CAD build for the part. Positions are in the model's coordinates, mm. Face numbers are marked on the shaded views. A direction names the side the tool comes from. Give positions to 0.01 mm unless a question says otherwise; leave off trailing zeros. Write each loop counter-clockwise with the first axis right and the second up, starting at its lowest first coordinate (ties: lowest second). Pieces come first, ordered by that corner, then holes. Notation, with made-up numbers: (-13.5, 39.5) -> (39.5, 39.5) arc R26 cw to (39.5, 57.5) -> close; hole circle Ø10 at (-31, 49). An arc over 180 degrees is marked (long way). Answer as a JSON object with one key per item and string values.
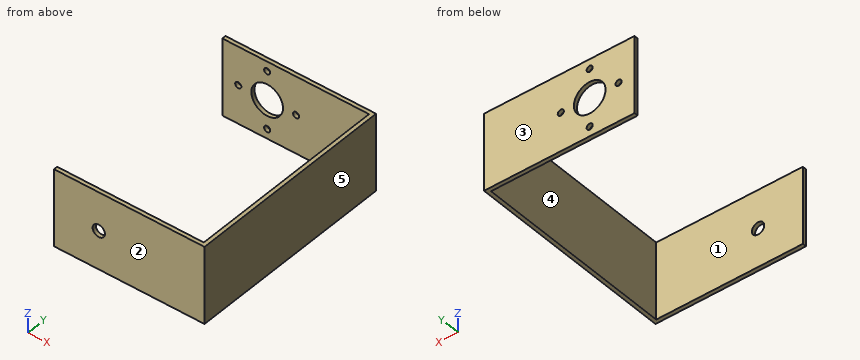
```python
from build123d import *

# Parameters (mm, degrees)
SKETCH_1_W          = 20
SKETCH_1_H          = 54.5
EXTRUDE_1_DEPTH     = 1
SKETCH_2_W          = 20
SKETCH_2_H          = 1
EXTRUDE_2_DEPTH     = 38
SKETCH_3_W          = 20
SKETCH_3_H          = 1
EXTRUDE_3_DEPTH     = 38
SKETCH_4_R          = 4.1
CUT_EXTRUDE_1_DEPTH = 1
SKETCH_5_R          = 0.79
CUT_EXTRUDE_2_DEPTH = 1
SKETCH_6_R          = 0.79
CUT_EXTRUDE_3_DEPTH = 1
SKETCH_7_R          = 0.79
CUT_EXTRUDE_4_DEPTH = 1
SKETCH_8_R          = 0.79
CUT_EXTRUDE_5_DEPTH = 1
SKETCH_9_R          = 1.6
CUT_EXTRUDE_6_DEPTH = 1


with BuildPart() as part:
    # ｽｹｯﾁ1 → ﾎﾞｽ - 押し出し1 (new body)
    with BuildSketch(Plane(origin=(0, 0, 0), x_dir=(0, 0, -1), z_dir=(1, 0, 0))):
        with Locations((10, 27.25)):
            Rectangle(SKETCH_1_W, SKETCH_1_H)
    extrude(amount=EXTRUDE_1_DEPTH)

    # ｽｹｯﾁ2 → ﾎﾞｽ - 押し出し2 (add)
    with BuildSketch(Plane.ZY):
        with Locations((-10, 54)):
            Rectangle(SKETCH_2_W, SKETCH_2_H)
    extrude(amount=EXTRUDE_2_DEPTH)

    # ｽｹｯﾁ3 → ﾎﾞｽ - 押し出し3 (add)
    with BuildSketch(Plane.ZY):
        with Locations((-10, 0.5)):
            Rectangle(SKETCH_3_W, SKETCH_3_H)
    extrude(amount=EXTRUDE_3_DEPTH)

    # ｽｹｯﾁ4 → ｶｯﾄ - 押し出し1 (cut)
    with BuildSketch(Plane(origin=(0, 54.5, 0), x_dir=(1, 0, 0), z_dir=(0, 1, 0))):
        with Locations((-26.39, 10)):
            Circle(SKETCH_4_R)
    extrude(amount=-CUT_EXTRUDE_1_DEPTH, mode=Mode.SUBTRACT)

    # ｽｹｯﾁ5 → ｶｯﾄ - 押し出し2 (cut)
    with BuildSketch(Plane(origin=(0, 54.5, 0), x_dir=(1, 0, 0), z_dir=(0, 1, 0))):
        with Locations((-33.88, 10)):
            Circle(SKETCH_5_R)
    extrude(amount=-CUT_EXTRUDE_2_DEPTH, mode=Mode.SUBTRACT)

    # ｽｹｯﾁ6 → ｶｯﾄ - 押し出し3 (cut)
    with BuildSketch(Plane(origin=(0, 54.5, 0), x_dir=(1, 0, 0), z_dir=(0, 1, 0))):
        with Locations((-18.9, 10)):
            Circle(SKETCH_6_R)
    extrude(amount=-CUT_EXTRUDE_3_DEPTH, mode=Mode.SUBTRACT)

    # ｽｹｯﾁ7 → ｶｯﾄ - 押し出し4 (cut)
    with BuildSketch(Plane(origin=(0, 54.5, 0), x_dir=(1, 0, 0), z_dir=(0, 1, 0))):
        with Locations((-26.39, 2.51)):
            Circle(SKETCH_7_R)
    extrude(amount=-CUT_EXTRUDE_4_DEPTH, mode=Mode.SUBTRACT)

    # ｽｹｯﾁ8 → ｶｯﾄ - 押し出し5 (cut)
    with BuildSketch(Plane(origin=(0, 54.5, 0), x_dir=(1, 0, 0), z_dir=(0, 1, 0))):
        with Locations((-26.39, 17.49)):
            Circle(SKETCH_8_R)
    extrude(amount=-CUT_EXTRUDE_5_DEPTH, mode=Mode.SUBTRACT)

    # ｽｹｯﾁ9 → ｶｯﾄ - 押し出し6 (cut)
    with BuildSketch(Plane(origin=(0, 0, 0), x_dir=(-1, 0, 0), z_dir=(0, -1, 0))):
        with Locations((26.39, 10)):
            Circle(SKETCH_9_R)
    extrude(amount=-CUT_EXTRUDE_6_DEPTH, mode=Mode.SUBTRACT)


solid = part.part
```
1) Wall check: probe 1 along Z at (x, y) = (-26.39, 53.9); probe 2 along Y at (x, z) = (-0.5, -5); probe 3 along X at (y, z) = (54.3, -10). Give the ranges that are in metal, low to high.
Model answer:
{"probe 1": "z = -20 to -18.28, -16.7 to -14.1, -5.9 to -3.3, -1.72 to 0", "probe 2": "y = 0 to 1, 53.5 to 54.5", "probe 3": "x = -38 to -34.67, -33.09 to -30.49, -22.29 to -19.69, -18.11 to 1"}
2) Slice it at D-D (y = 7). List the corners of the cut face in (x, z).
Model answer:
{"outline": "(0, -20) -> (1, -20) -> (1, 0) -> (0, 0) -> close"}
3) 3-axis set-ups, long thin cutter, end or side, ignore diameter. For the marked faces 1 and 2: which of +Z, -Z, +X, -X, +Y, -Y reach the whole face in a straight line?
Model answer:
{"face 1": "+Z, -Z, -X", "face 2": "+Z, -Z, +X, -X, -Y"}
4) Pin check, flat tip, straight feed: pin 1 (10 mm diameter, centred on y = 33, z = -11.5, fed in from -X). Stop position of the tip, or through.
Model answer:
{"pin 1": "stops at x = 0"}
5) Slice it at A-A (x = -18.9). List the corners of the cut face in (y, z).
Model answer:
{"outline": "(0, -20) -> (1, -20) -> (1, 0) -> (0, 0) -> close; (53.5, -20) -> (54.5, -20) -> (54.5, -10.79) -> (53.5, -10.79) -> close; (53.5, -9.21) -> (54.5, -9.21) -> (54.5, 0) -> (53.5, 0) -> close"}
6) Slice it at B-B (x = -4). List the corners of the cut face in (y, z).
Model answer:
{"outline": "(0, -20) -> (1, -20) -> (1, 0) -> (0, 0) -> close; (53.5, -20) -> (54.5, -20) -> (54.5, 0) -> (53.5, 0) -> close"}
7) Mould opens along Y. For the marked faces 3, 4 and 5 say: released by +Y, released by -Y, zero draft, split by the parting line, or undercut.
Model answer:
{"face 3": "released by +Y", "face 4": "undercut", "face 5": "zero draft"}
8) Slice it at C-C (z = -17.49). List the corners of the cut face in (x, y), then the cut area to 3 significant figures.
Model answer:
{"outline": "(-38, 0) -> (1, 0) -> (1, 54.5) -> (-25.6, 54.5) -> (-25.6, 53.5) -> (0, 53.5) -> (0, 1) -> (-38, 1) -> close; (-38, 53.5) -> (-27.18, 53.5) -> (-27.18, 54.5) -> (-38, 54.5) -> close", "area": "129 mm2"}
